```python
from build123d import *

# Parameters (mm, degrees)
SKETCH_1_W           = 50
SKETCH_1_H           = 25
SKETCH_1_R           = 2
EXTRUDE_3_DEPTH      = 20
SHELL_1_T            = -1.5
SKETCH_1_3_R         = 2
EXTRUDE_4_DEPTH      = 20
M2X0_4_3_D           = 1.6
M2X0_4_3_DEPTH       = 8
M2X0_4_3_CBORE_D     = 2
M2X0_4_3_CBORE_DEPTH = 4
M2X0_4_3_TIP         = 0.480688495


with BuildPart() as part:
    # Sketch 1 → Extrude 3 (new body)
    # profile 1 of 5: a face of its own
    with BuildSketch(Plane(origin=(0, 0, 0), x_dir=(1, 0, 0), z_dir=(0, 1, 0))):
        with Locations((25, 12.5)):
            Rectangle(SKETCH_1_W, SKETCH_1_H)
        with Locations((2.5, 2.5)):
            Circle(SKETCH_1_R, mode=Mode.SUBTRACT)
        with Locations((47.5, 2.5)):
            Circle(SKETCH_1_R, mode=Mode.SUBTRACT)
        with Locations((47.5, 22.5)):
            Circle(SKETCH_1_R, mode=Mode.SUBTRACT)
        with Locations((2.5, 22.5)):
            Circle(SKETCH_1_R, mode=Mode.SUBTRACT)
    # profile 2 of 5: a face of its own
    with BuildSketch(Plane(origin=(0, 0, 0), x_dir=(1, 0, 0), z_dir=(0, 1, 0))):
        with Locations((2.5, 22.5)):
            Circle(SKETCH_1_R)
    # profile 3 of 5: a face of its own
    with BuildSketch(Plane(origin=(0, 0, 0), x_dir=(1, 0, 0), z_dir=(0, 1, 0))):
        with Locations((47.5, 22.5)):
            Circle(SKETCH_1_R)
    # profile 4 of 5: a face of its own
    with BuildSketch(Plane(origin=(0, 0, 0), x_dir=(1, 0, 0), z_dir=(0, 1, 0))):
        with Locations((47.5, 2.5)):
            Circle(SKETCH_1_R)
    # profile 5 of 5: a face of its own
    with BuildSketch(Plane(origin=(0, 0, 0), x_dir=(1, 0, 0), z_dir=(0, 1, 0))):
        with Locations((2.5, 2.5)):
            Circle(SKETCH_1_R)
    extrude(amount=EXTRUDE_3_DEPTH)

    # Shell 1
    shell_1_openings = [part.faces().sort_by_distance(p)[0] for p in [
        (25, 20, -12.5),
    ]]
    offset(amount=SHELL_1_T, openings=shell_1_openings, kind=Kind.INTERSECTION)

    # Sketch 1_3 → Extrude 4 (add)
    with BuildSketch(Plane(origin=(0, 0, 0), x_dir=(1, 0, 0), z_dir=(0, 1, 0))):
        with Locations((2.5, 22.5)):
            Circle(SKETCH_1_3_R)
        with Locations((47.5, 22.5)):
            Circle(SKETCH_1_3_R)
        with Locations((47.5, 2.5)):
            Circle(SKETCH_1_3_R)
        with Locations((2.5, 2.5)):
            Circle(SKETCH_1_3_R)
    extrude(amount=EXTRUDE_4_DEPTH)

    # M2x0.4 _3
    with Locations(Plane(origin=(0, 20, 0), x_dir=(1, 0, 0), z_dir=(0, 1, 0))):
        with Locations((47.553254434, 22.471754376), (47.5, 2.5), (2.503648452, 22.471754376), (2.5, 2.5)):
            CounterBoreHole(M2X0_4_3_D / 2, M2X0_4_3_CBORE_D / 2, M2X0_4_3_CBORE_DEPTH, depth=M2X0_4_3_DEPTH)
            with Locations((0, 0, -(M2X0_4_3_DEPTH + M2X0_4_3_TIP / 2))):  # 118° drill point
                Cone(0, M2X0_4_3_D / 2, M2X0_4_3_TIP, mode=Mode.SUBTRACT)


solid = part.part
```
Design review of the part built by this model. Coordinates are the model's own, in mm. A direction names the side the tool comes from. Round coordinates to 2 decimals unless told otherwise and drop trailing zeros. Write each loop counter-clockwise with the first axis right and the second up, starting at its lowest first coordinate (ties: lowest second). Pieces come first, ordered by that corner, then holes. Notation, with made-up numbers: (8.5, 6) -> (29.5, 6) arc R33 ccw to (29.5, 43) -> close; hole circle Ø2 at (12, 83). An arc over 180 degrees is marked (long way). Write item = value, one per line. Start each with the question number.
1) Take a section at A-A, the plane y = 8.5. State the section outline as (x, z) points, plus the area to 3 significant figures.
2) Tool access review of faces 3 (the face through (25, 0, -13)), 4 (the face through (48.3, 14, -2.5)): name each direction out of +Z, -Z, +X, -X, +Y, -Y from which nothing blocks a thin tool from reaching the whole face with its end or side.
3) Take a section at D-D, the plane y = 18.5. State the section outline as (x, z) points.
4) Mouldability with a two-part tool opening along Z and no side actions: class faces 1 (the face through (2.578, 11.603, -22.589)), 2 (the face through (50, 10, -12)) as +Z half, -Z half, draft (parallel to the pull), parting line (faces both ways), or undercut.
5) Clearance check with a flat-ended pin moving along its axis: pin 1 (1 mm diameter, centred on x = 47.55, z = -22.47, fed in from +Y). State where the tip first meets the part, or that it passes through.
6) Wall thickness on probe 1 along Z at (x, y) = (2.5, 15); probe 2 along Z at (x, y) = (29, 4.75); probe 3 along X at (y, z) = (14, -17.5): over which ranges is each line inside the solid? List them lowest first. Write a range as from..to.
7) Take a section at C-C, the plane x = 15. State the section outline as (y, z) points, plus the area to 3 significant figures.
8) Take a section at B-B, the plane z = -10.5. State the section outline as (x, y) points, plus the area to 4 significant figures.
Results list:
q1.outline = (0, -25) -> (50, -25) -> (50, 0) -> (0, 0) -> close; hole (1.5, -20.77) arc R2 cw to (4.23, -23.5) -> (45.77, -23.5) arc R2 cw to (48.5, -20.77) -> (48.5, -4.23) arc R2 cw to (45.77, -1.5) -> (4.23, -1.5) arc R2 cw to (1.5, -4.23) -> close
q1.area = 248 mm²
q2.face_3 = +Z, -Z, +X, -X, -Y
q2.face_4 = +Y
q3.outline = (0, -25) -> (50, -25) -> (50, 0) -> (0, 0) -> close; hole circle Ø2 at (2.5, -22.47); hole (1.5, -20.77) arc R2 cw to (4.23, -23.5) -> (45.77, -23.5) arc R2 cw to (48.5, -20.77) -> (48.5, -4.23) arc R2 cw to (45.77, -1.5) -> (4.23, -1.5) arc R2 cw to (1.5, -4.23) -> close; hole circle Ø2 at (2.5, -2.5); hole circle Ø2 at (47.5, -2.5); hole circle Ø2 at (47.55, -22.47)
q4.face_1 = undercut
q4.face_2 = draft
q5.pin_1 = 11.82
q6.probe_1 = -25..-23.27, -21.67..-20.5, -4.5..-3.3, -1.7..0
q6.probe_2 = -25..-23.5, -1.5..0
q6.probe_3 = 0..1.5, 48.5..50
q7.outline = (0, -25) -> (20, -25) -> (20, -23.5) -> (1.5, -23.5) -> (1.5, -1.5) -> (20, -1.5) -> (20, 0) -> (0, 0) -> close
q7.area = 93.0 mm²
q8.outline = (0, 0) -> (50, 0) -> (50, 20) -> (48.5, 20) -> (48.5, 1.5) -> (1.5, 1.5) -> (1.5, 20) -> (0, 20) -> close
q8.area = 130.5 mm²
